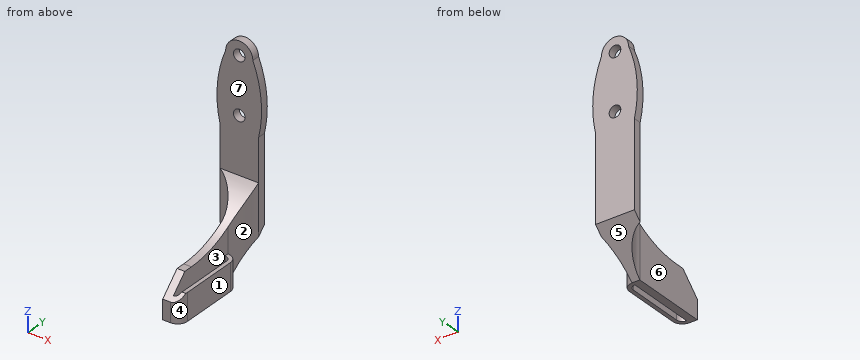
from build123d import *

# Parameters (mm, degrees)
SKETCH1_W           = 10
SKETCH1_H           = 22
SKETCH1_R           = 1.5
SKETCH1_R_2         = 3.5
BOSS_EXTRUDE1_DEPTH = 2
BOSS_EXTRUDE2_DEPTH = 10
CUT_EXTRUDE1_REACH  = 62.656
BOSS_EXTRUDE3_DEPTH = 7
CHAMFER1_SIZE       = 5


with BuildPart() as part:
    # Sketch1 → Boss-Extrude1 (new body)
    # profile 1 of 3: a face of its own
    with BuildSketch(Plane(origin=(0, 0, 0), x_dir=(1, 0, 0), z_dir=(0, 1, 0))):
        with Locations((0, 29)):
            Rectangle(SKETCH1_W, SKETCH1_H)
    # profile 2 of 3: a face of its own
    with BuildSketch(Plane(origin=(0, 0, 0), x_dir=(1, 0, 0), z_dir=(0, 1, 0))):
        with BuildLine():
            Line((5, 18), (-5, 18))
            ThreePointArc((-5, 18), (-5.636846209, 8.884429483), (-3.5, 0))
            ThreePointArc((-3.5, 0), (0, 3.5), (3.5, 0))
            ThreePointArc((3.5, 0), (5.636846209, 8.884429483), (5, 18))
        make_face()
        with Locations(Location((0, 14.5, 0), (0, 0, 270))):
            Circle(SKETCH1_R, mode=Mode.SUBTRACT)
    # profile 3 of 3: a face of its own
    with BuildSketch(Plane(origin=(0, 0, 0), x_dir=(1, 0, 0), z_dir=(0, 1, 0))):
        Circle(SKETCH1_R_2)
        with Locations(Location((0, 0, 0), (0, 0, 270))):
            Circle(SKETCH1_R, mode=Mode.SUBTRACT)
    extrude(amount=BOSS_EXTRUDE1_DEPTH)

    # Sketch2 → Boss-Extrude2 (add)
    with BuildSketch(Plane.ZY.offset(5)):
        with BuildLine():
            Line((-40, 2), (-50, -8))
            Line((-50, -8), (-50, -28))
            Line((-50, -28), (-40, -28))
            Line((-40, -28), (-40, -20.712315177))
            ThreePointArc((-40, -20.712315177), (-37.079402166, -8.986275778), (-29, 0))
            Line((-29, 0), (-40, 2))
        make_face()
    extrude(amount=-BOSS_EXTRUDE2_DEPTH)

    # Sketch3 → Cut-Extrude1 (cut, up to next)
    with BuildSketch(Plane(origin=(0, 0, -50), x_dir=(-1, 0, 0), z_dir=(0, 0, -1)), mode=Mode.PRIVATE) as cut_extrude1_sk1:
        with BuildLine():
            Line((-3, -8), (-3, -28))
            Line((-3, -28), (-5, -28))
            Line((-5, -28), (-5, 0))
            ThreePointArc((-5, 0), (-3.507577498, -3.876894374), (-3, -8))
        make_face()
    cut_extrude1_tool1 = extrude(cut_extrude1_sk1.sketch, amount=-CUT_EXTRUDE1_REACH, mode=Mode.PRIVATE) & part.part
    # Sketch3 → Cut-Extrude1 (cut, up to next)
    with BuildSketch(Plane(origin=(0, 0, -50), x_dir=(-1, 0, 0), z_dir=(0, 0, -1)), mode=Mode.PRIVATE) as cut_extrude1_sk2:
        with BuildLine():
            Line((-1, -8), (-1, -28))
            Line((-1, -28), (5, -28))
            Line((5, -28), (5, 0))
            ThreePointArc((5, 0), (0.666666667, -3), (-1, -8))
        make_face()
    cut_extrude1_tool2 = extrude(cut_extrude1_sk2.sketch, amount=-CUT_EXTRUDE1_REACH, mode=Mode.PRIVATE) & part.part
    add(cut_extrude1_tool1.solids().sort_by_distance((4.041628, -15.231137, -50))[0], mode=Mode.SUBTRACT)
    add(cut_extrude1_tool2.solids().sort_by_distance((-2.115152, -14.990475, -50))[0], mode=Mode.SUBTRACT)

    # Sketch4 → Boss-Extrude3 (add)
    with BuildSketch(Plane(origin=(0, 0, -50), x_dir=(-1, 0, 0), z_dir=(0, 0, -1))):
        with BuildLine():
            ThreePointArc((-3, -8), (-4.767766953, -8.732233047), (-5.5, -10.5))
            Line((-5.5, -10.5), (-5.5, -25.5))
            ThreePointArc((-5.5, -25.5), (-4.767766953, -27.267766953), (-3, -28))
            Line((-3, -28), (-3, -27))
            ThreePointArc((-3, -27), (-4.060660172, -26.560660172), (-4.5, -25.5))
            Line((-4.5, -25.5), (-4.5, -10.5))
            ThreePointArc((-4.5, -10.5), (-4.060660172, -9.439339828), (-3, -9))
            Line((-3, -9), (-3, -8))
        make_face()
    extrude(amount=-BOSS_EXTRUDE3_DEPTH)

    # Chamfer1
    # the kernel refuses this chamfer: 5 mm, written as the material it takes off along each edge
    with BuildSketch(Plane(origin=(-11.85841494, -28, -40), x_dir=(0, 0.9996219169112968, 0.027495876610586317), z_dir=(1, 0, 0))) as chamfer1_piece_1:
        Polygon((CHAMFER1_SIZE * 0.999621916911, -CHAMFER1_SIZE * 0.0274958766106), (-CHAMFER1_SIZE * 0.0274958766106, -CHAMFER1_SIZE * 0.999621916911), (0, 0), align=None)
    extrude(amount=27.71682988, mode=Mode.SUBTRACT)


solid = part.part
The model under review builds one solid part; all positions refer to its coordinate system, in mm. Face numbers are marked on the shaded views. A direction names the side the tool comes from. Give positions to 0.01 mm unless a question says otherwise; leave off trailing zeros. Order: outer loops, then holes, each group sorted by start corner. A loop starts at its lowest first (then second) coordinate and runs counter-clockwise, first axis right, second up. Notation, with made-up numbers: M 34.25,-37 L 51.25,-37 A21 cw 51.25,-17 Z; hole C 4,2.5 d3. An arc over 180 degrees is marked long. Use one line per item in the form item = value. Start each with the question number.
Item 1: We need section D-D on y = -2. Give the boundary of the cut face in (x, z).
Item 2: We need section A-A on z = -14.5. Give the boundary of the cut face in (x, y), plus the area to 3 significant figures.
Item 3: Insertion check: pin 1 Ø5.5 at (y, z) = (-15.5, -45.5) entering from +X; pin 2 Ø11 at (y, z) = (-15.5, -43) entering from -X; pin 3 Ø2 at (y, z) = (1, -29.5) entering from -X. Each pin has a flat end and moves straight along its axis. Give the tip position at first contact, or say it passes through.
Item 4: We need section B-B on y = -13. Give the boundary of the cut face in (x, z), plus the area to 3 significant figures.
Item 5: For the marked faces 5, 6 and 7, list the 3-axis set-ups (+Z, -Z, +X, -X, +Y, -Y) from which the entire face can be reached by the end or side of a thin tool; tool diameter is ignored.
Item 6: The part is to be moulded in two halves that separate along Y. For the marked faces 1, 2, 3 and 4, say which applies: pulls with the +Y half, pulls with the -Y half, needs draft (parallel to the pull), parting line crosses it, or undercut.
Item 7: We need section C-C on x = 2.25. Give the boundary of the cut face in (y, z).
Item 8: To check wall thickness, follow line 1 along X through (y, z) = (-18, -44); line 2 along Y through (x, z) = (-3.5, -15.5); line 3 along Y through (x, z) = (5, -46). State the ranges of each line that lie inside material, in increasing order. Write a range as from..to.
Completed:
q1.outline = M -1.55,-44 L 4.09,-44 L 4.09,-31.58 L -1.55,-31.58 Z
q2.outline = M -5.58,0 L -1.5,0 L -1.5,2 L -5.58,2 Z; M 1.5,0 L 5.58,0 L 5.58,2 L 1.5,2 Z
q2.area = 16.3 mm²
q3.pin_1 = 5.5
q3.pin_2 = 1
q3.pin_3 = -5
q4.outline = M 1,-50 L 3,-50 L 3,-38.78 L 1,-38.78 Z; M 4.5,-50 L 5.5,-50 L 5.5,-43 L 4.5,-43 Z
q4.area = 29.4 mm²
q5.face_5 = -Z, +X, -X, +Y
q5.face_6 = +Z, -Z, -X, -Y
q5.face_7 = +Z, +X, -X, -Y
q6.face_1 = needs draft
q6.face_2 = undercut
q6.face_3 = undercut
q6.face_4 = pulls with the -Y half
q7.outline = M -28,-50 L -8,-50 L 2,-40 L 2,2.68 L 0,2.68 L 0,-29 A25 cw -20.71,-40 L -23,-40 L -28,-45 Z
q8.line_1 = 1..3, 4.5..5.5
q8.line_2 = 0..2
q8.line_3 = -27..-9
